Work out the finished part from the listing and answer in its coordinate system (mm). Face numbers are marked on the shaded views. A direction names the side the tool comes from. Round coordinates to 2 decimals unless told otherwise and drop trailing zeros. Order: outer loops, then holes, each group sorted by start corner. A loop starts at its lowest first (then second) coordinate and runs counter-clockwise, first axis right, second up. Notation, with made-up numbers: (-2, 1.5) - (33, 1.5) arc R8 cw to (33, 11.5) - close; hole circle Ø4 at (8.25, 49.5). An arc over 180 degrees is marked (long way). One line per question, with ' | ' between items. Start each with the question number.
from build123d import *

# Parameters (mm, degrees)
SKETCH1_W            = 25.4
SKETCH1_H            = 28.575
BOSS_EXTRUDE1_DEPTH  = 3.175
SKETCH2_W            = 25.4
SKETCH2_H            = 3.175
BOSS_EXTRUDE2_DEPTH  = 25.4
SKETCH4_R            = 1.4097
CUT_EXTRUDE1_DEPTH   = 29.575
LPATTERN1_COUNT      = 2
LPATTERN1_PITCH      = 10.16
LPATTERN1_COUNT_DIR2 = 2
LPATTERN1_PITCH_DIR2 = 10.16


with BuildPart() as part:
    # Sketch1 → Boss-Extrude1 (new body)
    with BuildSketch(Plane.XY):
        Rectangle(SKETCH1_W, SKETCH1_H)
    extrude(amount=BOSS_EXTRUDE1_DEPTH)

    # Sketch2 → Boss-Extrude2 (add)
    with BuildSketch(Plane.XY.offset(3.175)):
        with Locations((0, -12.7)):
            Rectangle(SKETCH2_W, SKETCH2_H)
    extrude(amount=BOSS_EXTRUDE2_DEPTH)

    # Sketch4 → Cut-Extrude1 (cut, through all)
    with BuildSketch(Plane(origin=(0, 0, 0), x_dir=(-1, 0, 0), z_dir=(0, 0, -1))):
        with Locations((-5.08, 6.0325)):
            Circle(SKETCH4_R)
    cut_extrude1 = extrude(amount=-CUT_EXTRUDE1_DEPTH, mode=Mode.SUBTRACT)

    # LPattern1: Cut-Extrude1 2 × 2
    with Locations(*[(-j * LPATTERN1_PITCH_DIR2, -i * LPATTERN1_PITCH, 0) for i in range(LPATTERN1_COUNT) for j in range(LPATTERN1_COUNT_DIR2) if (i, j) != (0, 0)]):
        add(cut_extrude1, mode=Mode.SUBTRACT)


solid = part.part
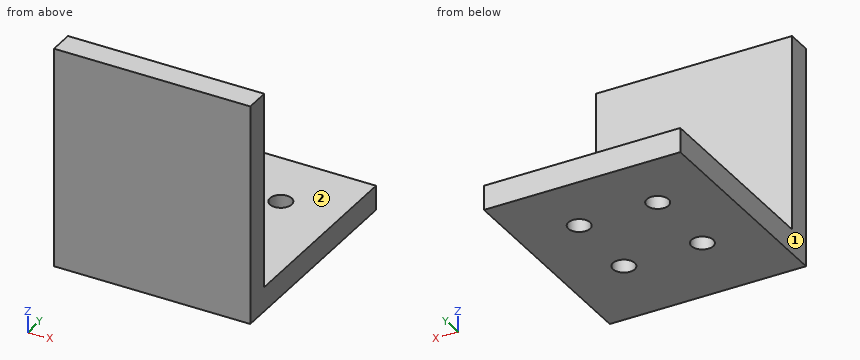
1) For the marked faces 1 and 2, determine the directions among +Z, -Z, +X, -X, +Y, -Y from which every point of the face is accessible in a straight line to the end or side of a thin tool.
2) Straight lines are drawn through the part: line 1 (Y direction, x = 5.08, z = 1.2); line 2 (Z direction, x = -2, y = 6.25) (3 decimals); line 3 (Y direction, x = -4.25, z = 27). For each, find the intervals that lie inside material, in ascending order.
3) Section A-A on x = -5.08 is taken. Give the vertices of the cut face in (y, z) (1 decimal).
4) Flat-ended cylindrical pins translate along their axes: pin 1 (5 mm diameter, centred on x = 1.5, z = 16, fed in from +Y); pin 2 (12.5 mm diameter, centred on x = -4.5, y = 0.5, fed in from +Z) (3 decimals). Find the tip coordinate at first contact, or state that the pin passes through.
5) Section C-C on z = 17.5 is taken. Give the vertices of the cut face in (x, y).
6) Section B-B on x = 11 is taken. Give the vertices of the cut face in (y, z) (1 decimal).
7) Section D-D on y = -7.75 is taken. Give the vertices of the cut face in (x, z) (3 decimals).
Recorded:
1) face 1: +Z, -Z, -X, +Y, -Y | face 2: +Z, +X, -X, +Y
2) line 1: y = -14.29 to -5.54, -2.72 to 4.62, 7.44 to 14.29 | line 2: z = 0 to 3.175 | line 3: y = -14.29 to -11.11
3) outline: (-14.3, 0) - (-5.5, 0) - (-5.5, 3.2) - (-11.1, 3.2) - (-11.1, 28.6) - (-14.3, 28.6) - close; (-2.7, 0) - (4.6, 0) - (4.6, 3.2) - (-2.7, 3.2) - close; (7.4, 0) - (14.3, 0) - (14.3, 3.2) - (7.4, 3.2) - close
4) pin 1: stops at y = -11.11 | pin 2: stops at z = 3.175
5) outline: (-12.7, -14.29) - (12.7, -14.29) - (12.7, -11.11) - (-12.7, -11.11) - close
6) outline: (-14.3, 0) - (14.3, 0) - (14.3, 3.2) - (-11.1, 3.2) - (-11.1, 28.6) - (-14.3, 28.6) - close
7) outline: (-12.7, 0) - (12.7, 0) - (12.7, 3.175) - (-12.7, 3.175) - close
